Autodesk Inventor part; units mm, degrees
ref_plane "YZ Plane" through (0, 0, 0) normal (1, 0, 0) x (0, 1, 0)
ref_plane "XZ Plane" through (0, 0, 0) normal (0, 1, 0) x (-1, 0, 0)
ref_plane "XY Plane" through (0, 0, 0) normal (0, 0, 1) x (1, 0, 0)
sketch "Boceto1" plane through (0, 0, 0) normal (0, 1, 0) x (-1, 0, 0)
  line L0 (0, 0) -> (0, -24)
  line L1 (10, 0) -> (0, 0)
  line L2 (55, -24) -> (55, 0)
  line L3 (55, 0) -> (10, 0)
  line L4 (0, -24) -> (0, -34)
  line L5 (0, -34) -> (55, -34)
  line L6 (55, -34) -> (55, -24)
  line L7 (0, 0) -> (5, 0)
  circle A0 centre (5, -6) radius 1.5
  circle A1 centre (5, -18) radius 1.5
  dimension "d0" = 24
  dimension "d4" = 10
  dimension "d7" = 5
extrude "Extrusión1" add sketch "Boceto1" along normal blind 8
sketch "Boceto2" plane through (0, 0, 0) normal (0, -1, 0) x (1, 0, 0)
  line L0 (0, 0) -> (0, -24.5)
  line L1 (0, 0) -> (0, -34)
  line L2 (0, -24.5) -> (-46, -24.5)
  line L3 (-55, -34) -> (-55, 0)
  line L4 (-55, -24.5) -> (-55, -34)
  line L5 (0, -34) -> (-55, -34)
  line L6 (0, -34) -> (-55, -34)
  line L7 (0, -34) -> (0, -24.5)
  line L8 (-55, 0) -> (0, 0)
  line L9 (-55, 0) -> (-46, 0)
  line L10 (-46, 0) -> (-46, -24.5)
  line L11 (-55, -24.5) -> (-55, 0)
  dimension "d15" = 24.5
  dimension "d16" = 9
extrude "Extrusión2" add sketch "Boceto2" along normal blind 45 contours L1 L5 L3 L8 L10 L2
sketch "Boceto3" plane through (0, 8, -34) normal (0, 0, -1) x (-1, 0, 0)
  circle A0 centre (5, -23) radius 1.5
  circle A1 centre (5, -40) radius 1.5
  point P0 (0, -8)
extrude "Extrusión3" cut sketch "Boceto3" against normal blind 45
fillet "Empalme1" radius 8 6 edges at (-27.5, 8, -34) (-55, -18.5, -34) (-55, 8, -17) (-27.5, -45, -34) (-55, -18.5, 0) (-55, -45, -17)
properties part number "Soporte_Brazo_IZQ"
Part model, mm, in its own coordinate system. A direction names the side the tool comes from. Give positions to 0.01 mm unless a question says otherwise; leave off trailing zeros. Loops run counter-clockwise (first coordinate to the right, second up) from the corner with the lowest first, then second, coordinate; pieces in that order, holes last. Notation, with made-up numbers: M 27.25,37 L 55.25,37 A20 cw 55.25,53 Z; hole C 25,-18 d10. An arc over 180 degrees is marked long. Return JSON: item names as keys, results as strings.
1) 3-axis set-ups, long thin cutter, end or side, ignore diameter. For faces 4 (the face through (-23, 0, -12)), 5 (the face through (-6.386, -15.575, -29.316)): which of +Z, -Z, +X, -X, +Y, -Y reach the whole face in a straight line?
Calculated:
{"face 4": "+Z, +X, -Y", "face 5": "+Z, -Z"}
2) Drill centre lines: line 1 (Y direction, x = -5, z = -26.5); line 2 (Z direction, x = -5, y = 3.5); line 3 (X direction, y = -15, z = -10.5). Where is each one in solid material? Low to high.
Calculated:
{"line 1": "y = -44.98 to -33.5, -30.5 to -16.5, -13.5 to 7.98", "line 2": "z = -33.19 to -19.5, -16.5 to -7.5, -4.5 to 0", "line 3": "x = -55 to -46"}
3) Saw through at A-A, the plane y = -32. List the corners of the cut face in (x, z).
Calculated:
{"outline": "M -55,-26 A8 ccw -47,-34 L -6.5,-34 L -6.5,-24.5 L -46,-24.5 L -46,0 L -47,0 A8 ccw -55,-8 Z; M -3.5,-34 L 0,-34 L 0,-24.5 L -3.5,-24.5 Z"}
4) Pull direction Z, two halves, no side cores. Call faces 1 (the face through (-23, -19, -34)), 2 (the face through (-6.386, 3.944, -5.425)), 3 (the face through (-55, -19, -17)): released by +Z, released by -Z, zero draft, split by the parting line, or undercut.
Calculated:
{"face 1": "released by -Z", "face 2": "undercut", "face 3": "zero draft"}
5) Saw through at B-B, the plane x = -5. List the corners of the cut face in (y, z).
Calculated:
{"outline": "M -45,-26 A8 ccw -37,-34 L -33.5,-34 L -33.5,-24.5 L -45,-24.5 Z; M -30.5,-34 L -16.5,-34 L -16.5,-24.5 L -30.5,-24.5 Z; M -13.5,-34 L 0,-34 A8 ccw 8,-26 L 8,-19.5 L 0,-19.5 L 0,-24.5 L -13.5,-24.5 Z; M 0,-16.5 L 8,-16.5 L 8,-7.5 L 0,-7.5 Z; M 0,-4.5 L 8,-4.5 L 8,0 L 0,0 Z"}
6) Saw through at D-D, the plane x = -12.5. List the corners of the cut face in (y, z), then the cut area to 3 significant figures.
Calculated:
{"outline": "M -45,-26 A8 ccw -37,-34 L 0,-34 A8 ccw 8,-26 L 8,0 L 0,0 L 0,-24.5 L -45,-24.5 Z", "area": "672 mm2"}
7) Saw through at C-C, the plane z = -18. List the corners of the cut face in (x, y).
Calculated:
{"outline": "M -55,-37 A8 ccw -47,-45 L -46,-45 L -46,0 L -6.5,0 L -6.5,8 L -47,8 A8 ccw -55,0 Z; M -3.5,0 L 0,0 L 0,8 L -3.5,8 Z"}
8) Flat gauge pins, fed straight in: pin 1 Ø12 at (x, z) = (-23, -13.5) entering from -Y; pin 2 Ø2 at (x, y) = (-13, -21) entering from +Z; pin 3 Ø7.5 at (y, z) = (-31.5, -10) entering from +X. Where does each tip first touch, or does it go through?
Calculated:
{"pin 1": "stops at y = 0", "pin 2": "stops at z = -24.5", "pin 3": "stops at x = -46"}
